Design review of the part shown in the three views and the two pictorial views. Dimensions are in mm from the part's minimum x, y and z. Round coordinates to 2 decimals unless told otherwise and drop trailing zeros. Write each loop counter-clockwise with the first axis right and the second up, starting at its lowest first coordinate (ties: lowest second). Pieces come first, ordered by that corner, then holes. Notation, with made-up numbers: (-6, 70) - (50, 70) arc R32 ccw to (50, 98) - close; hole circle Ø9 at (-20, -34). An arc over 180 degrees is marked (long way). Use one line per item in the form item = value.
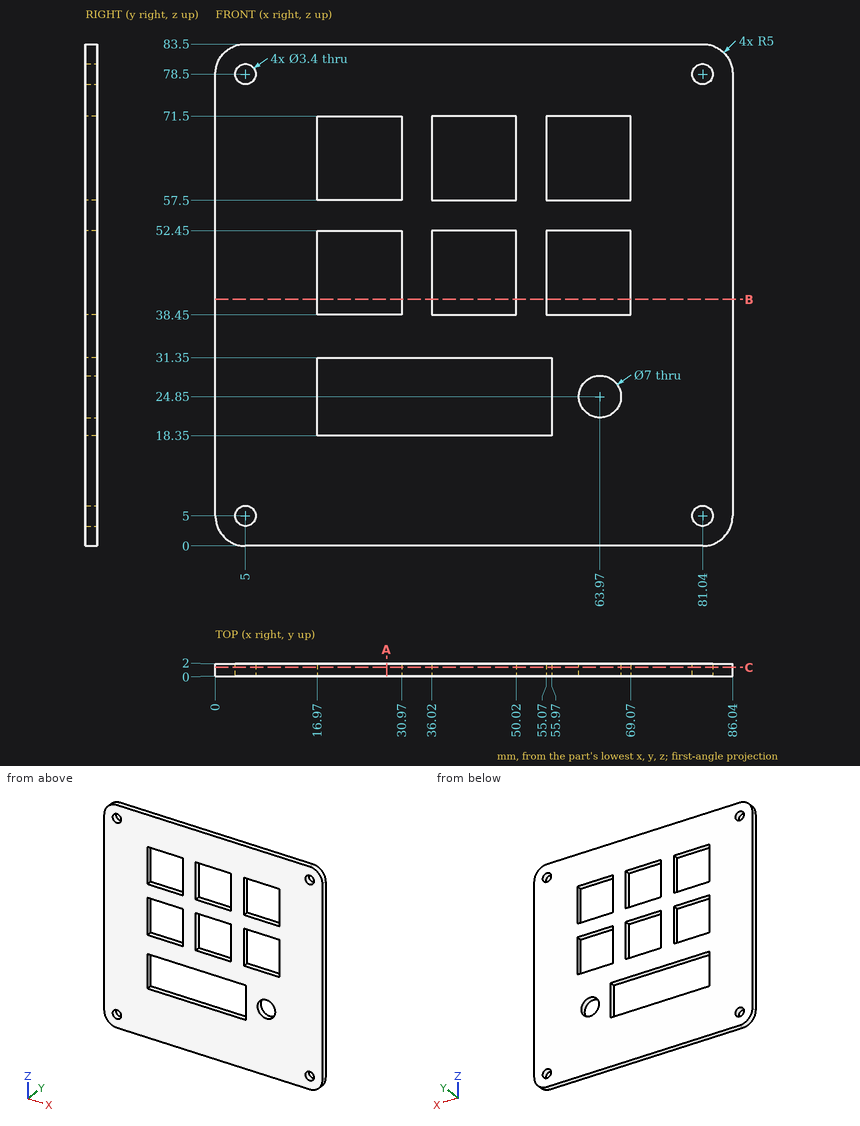
Q1. We need section B-B on z = 41. Write out the cut boundary in (x, y).
Calculated:
outline = (0, 0) - (16.97, 0) - (16.97, 2) - (0, 2) - close; (30.97, 0) - (36.02, 0) - (36.02, 2) - (30.97, 2) - close; (50.02, 0) - (55.07, 0) - (55.07, 2) - (50.02, 2) - close; (69.07, 0) - (86.04, 0) - (86.04, 2) - (69.07, 2) - close
Q2. We need section C-C on y = 1.45. State how many separate pieces and enclosed holes the cut face has, then the cut area to 3 significant figures.
Calculated:
separate_pieces = 1
enclosed_holes = 12
area = 5,410 mm2
Q3. For P1, Ø12, axis at x = 45.5, z = 20.5, coming from the -Y side; P2, Ø3, axis at x = 39, z = 42.5, coming from the +Y side, all flat-tipped, find the tip position at first contact; note any pin that passes through.
Calculated:
P1 = 0
P2 = through
Q4. We need section A-A on x = 28.5. Write out the cut boundary in (y, z).
Calculated:
outline = (0, 0) - (2, 0) - (2, 18.35) - (0, 18.35) - close; (0, 31.35) - (2, 31.35) - (2, 38.45) - (0, 38.45) - close; (0, 52.45) - (2, 52.45) - (2, 57.5) - (0, 57.5) - close; (0, 71.5) - (2, 71.5) - (2, 83.5) - (0, 83.5) - close
Q5. To check wall thickness, follow line 1 along X through (y, z) = (1.7, 49.5); line 2 along Z through (x, y) = (69, 1.35); line 3 along Z through (x, y) = (38, 0.95). State the ranges of each line that lie inside material, in increasing order. Write a range as from..to.
Calculated:
line_1 = 0..16.97, 30.97..36.02, 50.02..55.07, 69.07..86.04
line_2 = 0..38.45, 52.45..57.5, 71.5..83.5
line_3 = 0..18.35, 31.35..38.45, 52.45..57.5, 71.5..83.5
